The model under review builds one solid part; all positions refer to its coordinate system, in mm. Face numbers are marked on the shaded views. A direction names the side the tool comes from. Round coordinates to 2 decimals unless told otherwise and drop trailing zeros. Order: outer loops, then holes, each group sorted by start corner. A loop starts at its lowest first (then second) coordinate and runs counter-clockwise, first axis right, second up. Notation, with made-up numbers: (-13, -0.75) - (27, -0.75) arc R20 ccw to (27, 6.25) - close; hole circle Ø6 at (83, 58). An arc over 180 degrees is marked (long way). One line per question, with ' | ' between items. Start each with the question number.
Item 1: Add section D-D on z = -1.5. State the section outline as (x, y) points (3 decimals), and give its area (3 significant figures).
Item 2: Insertion check: pin 1 Ø1.5 at (y, z) = (8, 6.5) entering from -X; pin 2 Ø3 at (x, z) = (0.5, 7) entering from -Y; pin 3 Ø1.4 at (y, z) = (4.5, 7.5) entering from -X. Each pin has a flat end and moves straight along its axis. Give the tip position at first contact, or say it passes through.
Item 3: Add section C-C on y = 7.25. State the section outline as (x, z) points (3 decimals), and give its area (3 significant figures).
Item 4: Add section B-B on z = 5. State the section outline as (x, y) points (3 decimals).
Item 5: Tool access review of the marked faces 4, 5, 6, 7 and 8: name each direction out of +Z, -Z, +X, -X, +Y, -Y from which nothing blocks a thin tool from reaching the whole face with its end or side.
Item 6: For L1, parallel to Y at x = 0, z = 8.1 (3 decimals); L2, parallel to Y at x = -0.7, z = 6.25; L3, parallel to Y at x = 0.95, z = 6.75, list the stretches that pass through material, from the lowest coordinate up. Write a range as [from, to].
Item 7: Add section A-A on x = 0. State the section outline as (y, z) points (3 decimals).
Item 8: Draft analysis for pull direction X (two halves, no side actions). For the marked faces 1, 2 and 3, state which applies: +X half, -X half, draft (parallel to the pull), parting line (faces both ways), or undercut.
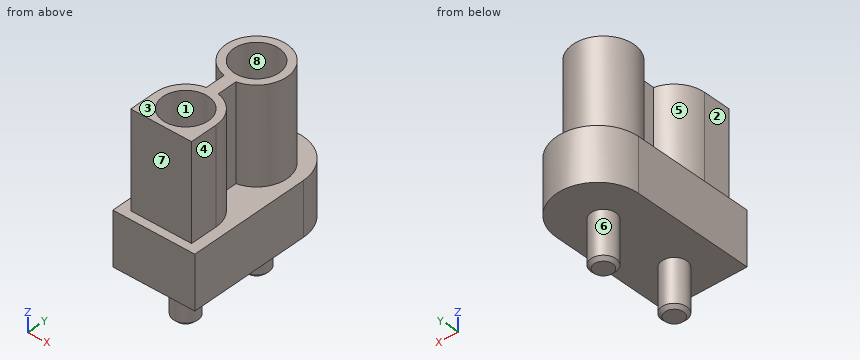
from build123d import *

# Parameters (mm, degrees)
SALIENTE_EXTRUIR1_DEPTH = 3.35
CROQUIS2_R              = 0.775
SALIENTE_EXTRUIR2_DEPTH = 2.9
CHAFL_N1_SIZE           = 0.2
CROQUIS3_R              = 1.425
SALIENTE_EXTRUIR3_DEPTH = 6


with BuildPart() as part:
    # Croquis1 → Saliente-Extruir1 (new body)
    with BuildSketch(Plane.XY):
        with BuildLine():
            Line((-2.575, 7.655), (-2.575, 0))
            Line((-2.575, 0), (2.575, 0))
            Line((2.575, 0), (2.575, 7.655))
            ThreePointArc((2.575, 7.655), (0, 10.23), (-2.575, 7.655))
        make_face()
    extrude(amount=SALIENTE_EXTRUIR1_DEPTH)

    # Croquis2 → Saliente-Extruir2 (add)
    with BuildSketch(Plane(origin=(0, 0, 0), x_dir=(-1, 0, 0), z_dir=(0, 0, -1))):
        with Locations((0, 7.25)):
            Circle(CROQUIS2_R)
        with Locations((0, 2.25)):
            Circle(CROQUIS2_R)
    extrude(amount=SALIENTE_EXTRUIR2_DEPTH)

    # Chaflán1
    chafl_n1_edges = [part.edges().sort_by_distance(p)[0] for p in [
        (0.775, 7.25, -2.9),
        (0.775, 2.25, -2.9),
    ]]
    chamfer(chafl_n1_edges, length=CHAFL_N1_SIZE)

    # Croquis3 → Saliente-Extruir3 (add)
    with BuildSketch(Plane.XY.offset(3.35)):
        with BuildLine():
            Line((-1.91, 2.25), (-1.91, 0.51859855))
            Line((-1.91, 0.51859855), (1.91, 0.51859855))
            Line((1.91, 0.51859855), (1.91, 2.25))
            ThreePointArc((1.91, 2.25), (1.47721867, 3.460753897), (0.375, 4.122825406))
            Line((0.375, 4.122825406), (0.375, 5.377174594))
            ThreePointArc((0.375, 5.377174594), (0, 9.16), (-0.375, 5.377174594))
            Line((-0.375, 5.377174594), (-0.375, 4.122825406))
            ThreePointArc((-0.375, 4.122825406), (-1.47721867, 3.460753897), (-1.91, 2.25))
        make_face()
        with Locations((0, 2.25)):
            Circle(CROQUIS3_R, mode=Mode.SUBTRACT)
        with Locations((0, 7.25)):
            Circle(CROQUIS3_R, mode=Mode.SUBTRACT)
    extrude(amount=SALIENTE_EXTRUIR3_DEPTH)


solid = part.part
Determined:
1) outline: circle Ø1.55 at (0, 2.25); circle Ø1.55 at (0, 7.25) | area: 3.77 mm2
2) pin 1: x = -1.91 | pin 2: y = 0.52 | pin 3: x = -1.12
3) outline: (-2.575, 0) - (-0.775, 0) - (-0.775, -2.7) - (-0.575, -2.9) - (0.575, -2.9) - (0.775, -2.7) - (0.775, 0) - (2.575, 0) - (2.575, 3.35) - (1.91, 3.35) - (1.91, 9.35) - (1.425, 9.35) - (1.425, 3.35) - (-1.425, 3.35) - (-1.425, 9.35) - (-1.91, 9.35) - (-1.91, 3.35) - (-2.575, 3.35) - close | area: 27.5 mm2
4) outline: (-1.91, 0.519) - (1.91, 0.519) - (1.91, 2.25) arc R1.91 ccw to (0.375, 4.123) - (0.375, 5.377) arc R1.91 ccw (long way) to (-0.375, 5.377) - (-0.375, 4.123) arc R1.91 ccw to (-1.91, 2.25) - close; hole circle Ø2.85 at (0, 2.25); hole circle Ø2.85 at (0, 7.25)
5) face 4: +Z, +X, +Y, -Y | face 5: +Z, -X | face 6: -Z | face 7: +Z, +X, -X, -Y | face 8: +Z
6) L1: [0.519, 0.825], [3.675, 5.825], [8.675, 9.16] | L2: [0.52, 1.01], [3.49, 4.03], [5.47, 6.01], [8.49, 9.03] | L3: [0.52, 1.19], [3.31, 3.91], [5.59, 6.19], [8.31, 8.91]
7) outline: (0, 0) - (1.475, 0) - (1.475, -2.7) - (1.675, -2.9) - (2.825, -2.9) - (3.025, -2.7) - (3.025, 0) - (6.475, 0) - (6.475, -2.7) - (6.675, -2.9) - (7.825, -2.9) - (8.025, -2.7) - (8.025, 0) - (10.23, 0) - (10.23, 3.35) - (9.16, 3.35) - (9.16, 9.35) - (8.675, 9.35) - (8.675, 3.35) - (5.825, 3.35) - (5.825, 9.35) - (3.675, 9.35) - (3.675, 3.35) - (0.825, 3.35) - (0.825, 9.35) - (0.519, 9.35) - (0.519, 3.35) - (0, 3.35) - close
8) face 1: undercut | face 2: -X half | face 3: draft
